Geometry: final body of the model. Coordinates: model frame, mm. Face numbers are marked on the shaded views. A direction names the side the tool comes from. Give positions to 0.01 mm unless a question says otherwise; leave off trailing zeros. Loops run counter-clockwise (first coordinate to the right, second up) from the corner with the lowest first, then second, coordinate; pieces in that order, holes last.
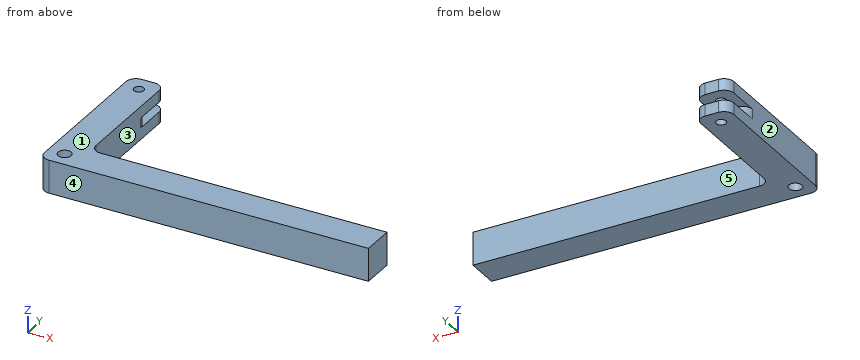
from build123d import *

# Parameters (mm, degrees)
SKETCH1_R             = 2
BOSS_EXTRUDE1_DEPTH   = 10
SKETCH2_W             = 10
SKETCH2_H             = 3
CUT_EXTRUDE1_DEPTH    = 10
F_3_0MM_DOWEL_HOLE1_D = 3
FILLET2_R             = 3


with BuildPart() as part:
    # Sketch1 → Boss-Extrude1 (new body)
    with BuildSketch(Plane.XY):
        Polygon((0, 0), (100, 0), (100, 10), (10, 10), (10, 50), (0, 50), align=None)
        with Locations((5, 5)):
            Circle(SKETCH1_R, mode=Mode.SUBTRACT)
    extrude(amount=BOSS_EXTRUDE1_DEPTH)

    # Sketch2 → Cut-Extrude1 (cut)
    with BuildSketch(Plane(origin=(0, 50, 0), x_dir=(1, 0, 0), z_dir=(0, 1, 0))):
        with Locations((5, -5)):
            Rectangle(SKETCH2_W, SKETCH2_H)
    extrude(amount=-CUT_EXTRUDE1_DEPTH, mode=Mode.SUBTRACT)

    # Ø3.0mm Dowel Hole1 (through all)
    with Locations(Plane(origin=(0, 0, 0), x_dir=(1, 0, 0), z_dir=(0, 0, -1))):
        with Locations((5, -45)):
            Hole(F_3_0MM_DOWEL_HOLE1_D / 2)

    # Fillet2
    fillet2_edges = [part.edges().sort_by_distance(p)[0] for p in [
        (0, 50, 8.25),
        (10, 50, 8.25),
        (10, 10, 5),
        (0, 0, 5),
        (0, 50, 1.75),
        (10, 50, 1.75),
        (0, 40, 5),
        (10, 40, 5),
    ]]
    fillet(fillet2_edges, radius=FILLET2_R)


solid = part.part
Item 1: Ray query, probe 1 along Y at (x, z) = (5, 1.4); probe 2 along Y at (x, z) = (5, 5.75); probe 3 along Y at (x, z) = (28.5, 5.25). Return the intervals inside material, ascending.
Values follow:
probe 1: y = 0 to 3, 7 to 43.5, 46.5 to 50
probe 2: y = 0 to 3, 7 to 40
probe 3: y = 0 to 10
Item 2: Pin query (flat end, axial travel): pin 1 (4 mm diameter, centred on x = 53, z = 5, fed in from +Y); pin 2 (0.9 mm diameter, centred on x = 4, z = 5, fed in from +Y); pin 3 (4 mm diameter, centred on x = 5, y = 45, fed in from -Z). Return the tip coordinate at first contact, or that it passes through.
Values follow:
pin 1: stops at y = 10
pin 2: stops at y = 40
pin 3: stops at z = 0
Item 3: Section query C-C on z = 1. Return loops of the section in (x, y), plus the area to 3 significant figures.
Values follow:
outline: (0, 3) arc R3 ccw to (3, 0) - (100, 0) - (100, 10) - (13, 10) arc R3 cw to (10, 13) - (10, 47) arc R3 ccw to (7, 50) - (3, 50) arc R3 ccw to (0, 47) - close; hole circle Ø4 at (5, 5); hole circle Ø3 at (5, 45)
area: 1,380 mm2
Item 4: Draft query along X for the marked faces 1, 2 and 3. Return one class per face: +X half, -X half, draft (parallel to the pull), parting line (faces both ways), or undercut.
Values follow:
face 1: draft
face 2: -X half
face 3: +X half
Item 5: Section query D-D on y = 45. Return loops of the section in (x, z).
Values follow:
outline: (0, 0) - (3.5, 0) - (3.5, 3.5) - (0, 3.5) - close; (0, 6.5) - (3.5, 6.5) - (3.5, 10) - (0, 10) - close; (6.5, 0) - (10, 0) - (10, 3.5) - (6.5, 3.5) - close; (6.5, 6.5) - (10, 6.5) - (10, 10) - (6.5, 10) - close
Item 6: Section query A-A on x = 5. Return loops of the section in (y, z), plus the area to 3 significant figures.
Values follow:
outline: (0, 0) - (3, 0) - (3, 10) - (0, 10) - close; (7, 0) - (43.5, 0) - (43.5, 3.5) - (40, 3.5) - (40, 6.5) - (43.5, 6.5) - (43.5, 10) - (7, 10) - close; (46.5, 0) - (50, 0) - (50, 3.5) - (46.5, 3.5) - close; (46.5, 6.5) - (50, 6.5) - (50, 10) - (46.5, 10) - close
area: 409 mm2
Item 7: Set-up query: the marked faces 4 and 5. Return all of +Z, -Z, +X, -X, +Y, -Y with unobstructed straight access to the full face (end or side cutting, diameter ignored); none if empty.
Values follow:
face 4: +Z, -Z, +X, -X, -Y
face 5: +Z, -Z, +X, +Y
Item 8: Section query B-B on y = 5. Return loops of the section in (x, z), plus the area to 3 significant figures.
Values follow:
outline: (0, 0) - (3, 0) - (3, 10) - (0, 10) - close; (7, 0) - (100, 0) - (100, 10) - (7, 10) - close
area: 960 mm2
